Geometry: final body of the model. Coordinates: model frame, mm. Face numbers are marked on the shaded views. A direction names the side the tool comes from. Round coordinates to 2 decimals unless told otherwise and drop trailing zeros. Order: outer loops, then holes, each group sorted by start corner. A loop starts at its lowest first (then second) coordinate and runs counter-clockwise, first axis right, second up. Notation, with made-up numbers: M 72.5,-0.5 L 76.5,-0.5 A27 cw 76.5,28.5 Z; hole C 44,-18 d2. An arc over 180 degrees is marked long. Put each result on its own line as item: value. Start each with the question number.
1) Material intervals for probe 1 along Y at (x, z) = (-41, 37.5); probe 2 along X at (y, z) = (-29, 45); probe 3 along Z at (x, y) = (-56, -21.5), sorted ascending. Write a range as [from, to].
2) First-contact query: P1, Ø2, axis at x = -59.5, y = 30.08, coming from the +Z side; P2, Ø10, axis at x = 10, y = -26.5, coming from the +Z side; P3, Ø4.5, axis at x = 28.5, y = 29.94, coming from the -Z side. Flat tips, straight axial feed; report the tip coordinate or a pass-through.
3) Section A-A, the plane z = 20.5. Return loops of the section in (x, y), then the cut area to 3 significant figures.
4) Section C-C, the plane x = -20. Return loops of the section in (y, z).
5) Access query for the marked faces 1 and 2. Directions: +Z, -Z, +X, -X, +Y, -Y. A direction counts if a zero-diameter tool reaches every point of the face in a straight line with its end or side. Return the directions, or none.
6) Section B-B, the plane y = 4. Return loops of the section in (x, z), then the cut area to 3 significant figures.
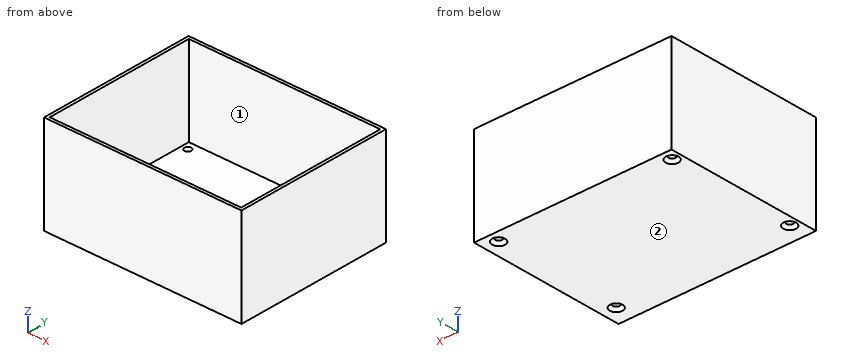
from build123d import *

# Parameters (mm, degrees)
SKETCH004_W     = 100
SKETCH004_H     = 80
SKETCH004_R     = 1.75
PAD003_DEPTH    = 4.5
CHAMFER001_SIZE = 1.5
SKETCH003_W     = 100
SKETCH003_H     = 80
SKETCH003_W_2   = 97
SKETCH003_H_2   = 77
PAD002_DEPTH    = 45


with BuildPart() as part:
    # Sketch004 → Pad003 (new body)
    with BuildSketch(Plane.XY):
        with Locations((-14.266246, -4.330319)):
            Rectangle(SKETCH004_W, SKETCH004_H)
        with Locations((-59.499317, 30.08403)):
            Circle(SKETCH004_R, mode=Mode.SUBTRACT)
        with Locations((28.500683, 29.937424)):
            Circle(SKETCH004_R, mode=Mode.SUBTRACT)
        with Locations((-59.584126, -34.915915)):
            Circle(SKETCH004_R, mode=Mode.SUBTRACT)
        with Locations((28.415874, -35.062521)):
            Circle(SKETCH004_R, mode=Mode.SUBTRACT)
    extrude(amount=PAD003_DEPTH)

    # Chamfer001
    chamfer001_edges = [part.edges().sort_by_distance(p)[0] for p in [
        (-61.334126, -34.915915, 0),
        (26.665874, -35.062521, 0),
        (26.750683, 29.937424, 0),
        (-61.249317, 30.08403, 0),
    ]]
    chamfer(chamfer001_edges, length=CHAMFER001_SIZE)

    # Sketch003 (on Face3 of Chamfer001) → Pad002 (join)
    with BuildSketch(Plane.XY.offset(4.5)):
        with Locations((-14.266246, -4.330319)):
            Rectangle(SKETCH003_W, SKETCH003_H)
        with Locations((-14.266246, -4.330319)):
            Rectangle(SKETCH003_W_2, SKETCH003_H_2, mode=Mode.SUBTRACT)
    extrude(amount=PAD002_DEPTH)


solid = part.part
Result sheet:
1. probe 1: y = [-44.33, -42.83], [34.17, 35.67]
1. probe 2: x = [-64.27, -62.77], [34.23, 35.73]
1. probe 3: z = [0, 4.5]
2. P1: passes through
2. P2: stops at z = 4.5
2. P3: stops at z = 1
3. outline: M -64.27,-44.33 L 35.73,-44.33 L 35.73,35.67 L -64.27,35.67 Z; hole M -62.77,-42.83 L 34.23,-42.83 L 34.23,34.17 L -62.77,34.17 Z
3. area: 531 mm2
4. outline: M -44.33,0 L 35.67,0 L 35.67,49.5 L 34.17,49.5 L 34.17,4.5 L -42.83,4.5 L -42.83,49.5 L -44.33,49.5 Z
5. face 1: +Z
5. face 2: -Z, +X, -X, +Y, -Y
6. outline: M -64.27,0 L 35.73,0 L 35.73,49.5 L 34.23,49.5 L 34.23,4.5 L -62.77,4.5 L -62.77,49.5 L -64.27,49.5 Z
6. area: 585 mm2
